from build123d import *
from build123d import SkipClean  # not in build123d's __all__

# Parameters (mm, degrees)
F0_W                   = 3
F0_H                   = 25.3
F0_W_2                 = 30.5
F1_DEPTH               = 3
F2_DEPTH               = 5
F3_R                   = 1.35
F4_DEPTH               = 500
F7_SIZE                = 5
F8_R                   = 1.35
F9_DEPTH               = 1
F10_W                  = 15
F10_H                  = 15
F11_DEPTH              = 3
F12_W                  = 4
F12_H                  = 5
F13_DEPTH              = 3
F12_W_2                = 4.5
F12_H_2                = 5.5
F14_DEPTH              = 25
F15_DEPTH              = 5
F16_R                  = 3.75
F17_DEPTH              = 2
F20_D                  = 3
F20_DEPTH              = 3
F20_CBORE_D            = 3
F20_CBORE_DEPTH        = 3
F20_TIP                = 0.9012909285
F20_ON_F19_D           = 3
F20_ON_F19_DEPTH       = 3
F20_ON_F19_CBORE_D     = 3
F20_ON_F19_CBORE_DEPTH = 3
F20_ON_F19_TIP         = 0.9012909285
F21_SIZE               = 10
F22_DEPTH              = 1
F23_SIZE               = 4.99999


# Not quite as in the source:
# - a fillet or chamfer is up to 0.001 mm smaller than in the source, because OpenCascade refuses the exact size


with BuildPart() as f1:
    # F0 (on Top) → F1 (new body)
    with BuildSketch(Plane.XY):
        with Locations((16.75, 0)):
            Rectangle(F0_W, F0_H)
        Rectangle(F0_W_2, F0_H)
        with Locations((-16.75, 0)):
            Rectangle(F0_W, F0_H)
    extrude(amount=F1_DEPTH)

    # F0 (on Top) → F2 (join)
    with BuildSketch(Plane.XY):
        with Locations((16.75, 0)):
            Rectangle(F0_W, F0_H)
        with Locations((-16.75, 0)):
            Rectangle(F0_W, F0_H)
    extrude(amount=-F2_DEPTH)

    # F3 (on face) → F4 (cut, symmetric)
    with BuildSketch(Plane(origin=(15.25, 0, 0), x_dir=(0, -1, 0), z_dir=(-1, 0, 0))):
        with BuildLine():
            Line((12.65, -4.15), (12.65, -1.45))
            ThreePointArc((12.65, -1.45), (11.3, -2.8), (12.65, -4.15))
        make_face()
        with Locations((-4.35, -2.8)):
            Circle(F3_R)
    extrude(amount=F4_DEPTH, both=True, mode=Mode.SUBTRACT)

    # F6: F1 across plane


with BuildPart() as f1_1:
    add(f1.part, clean=False)
    with SkipClean():  # cleaning this boolean's faces spoils the solid; the shape is the same uncleaned
        add(f1.part.mirror(Plane.XZ.offset(12.65)), clean=False)

    # F7
    f7_edges = [f1_1.edges().sort_by_distance(p)[0] for p in [
        (-16.75, 12.65, -5),
        (16.75, 12.65, -5),
        (16.75, -37.95, -5),
        (-16.75, -37.95, -5),
    ]]
    chamfer(f7_edges, length=F7_SIZE)

    # F8 (on face) → F9 (cut)
    with BuildSketch(Plane(origin=(-18.25, 0, 0), x_dir=(0, -1, 0), z_dir=(-1, 0, 0))):
        with BuildLine():
            Line((12.65, 0), (-12.65, 0))
            Line((-12.65, 0), (-7.65, -5))
            Line((-7.65, -5), (12.65, -5))
            Line((12.65, -5), (12.65, -4.15))
            ThreePointArc((12.65, -4.15), (11.3, -2.8), (12.65, -1.45))
            Line((12.65, -1.45), (12.65, 0))
        make_face()
        with Locations((-4.35, -2.8)):
            Circle(F8_R, mode=Mode.SUBTRACT)
        with BuildLine():
            Line((37.95, 0), (12.65, 0))
            Line((12.65, 0), (12.65, -1.45))
            ThreePointArc((12.65, -1.45), (14, -2.8), (12.65, -4.15))
            Line((12.65, -4.15), (12.65, -5))
            Line((12.65, -5), (32.95, -5))
            Line((32.95, -5), (37.95, 0))
        make_face()
        with Locations((29.65, -2.8)):
            Circle(F8_R, mode=Mode.SUBTRACT)
    extrude(amount=-F9_DEPTH, mode=Mode.SUBTRACT)

    # F10 (on Top) → F11 (join)
    with BuildSketch(Plane.XY):
        with Locations((-10.75, -45.45)):
            Rectangle(F10_W, F10_H)
        with Locations((-10.75, 20.15)):
            Rectangle(F10_W, F10_H)
    extrude(amount=F11_DEPTH)

    # F12 (on face) → F13 (join)
    with BuildSketch(Plane(origin=(0, 0, 0), x_dir=(1, 0, 0), z_dir=(0, 0, -1))):
        with Locations((-20.25, 50.45)):
            Rectangle(F12_W, F12_H)
    extrude(amount=-F13_DEPTH)

    # F12 (on face) → F14 (cut)
    with BuildSketch(Plane(origin=(0, 0, 0), x_dir=(1, 0, 0), z_dir=(0, 0, -1))):
        with Locations((-16, -24.9)):
            Rectangle(F12_W_2, F12_H_2)
    extrude(amount=-F14_DEPTH, mode=Mode.SUBTRACT)

    # F15 (add): faces of the model
    f15_faces = [f1_1.faces().sort_by_distance(p)[0] for p in [
        (-18.25, 0, 1.5),
        (-18.25, -25.3, 1.5),
        (-18.25, -42.95, 1.5),
        (-18.25, 17.4, 1.5),
        (-22.25, -50.45, 1.5),
        (-13.75, 24.9, 1.5),
    ]]
    extrude(f15_faces, amount=F15_DEPTH)

    # F16 (on face) → F17 (join)
    with BuildSketch(Plane(origin=(0, 0, 0), x_dir=(1, 0, 0), z_dir=(0, 0, -1))):
        with BuildLine():
            Line((-13.75, -22.15), (-18, -22.15))
            ThreePointArc((-18, -22.15), (-16.7185522073, -24.9728974477), (-13.75, -25.8665171868))
            Line((-13.75, -25.8665171868), (-13.75, -22.15))
        make_face()
        with BuildLine():
            ThreePointArc((-13.75, -25.8665171868), (-11.4271025523, -24.6185522073), (-10.5, -22.15))
            ThreePointArc((-10.5, -22.15), (-14.25, -18.4), (-18, -22.15))
            Line((-18, -22.15), (-13.75, -22.15))
            Line((-13.75, -22.15), (-13.75, -25.8665171868))
        make_face()
        with Locations((-14.25, 47.45)):
            Circle(F16_R)
    extrude(amount=F17_DEPTH)

    # F20
    with Locations(Plane(origin=(0, 0, -2), x_dir=(1, 0, 0), z_dir=(0, 0, -1))):
        with Locations((-14.25, 47.45)):
            CounterBoreHole(F20_D / 2, F20_CBORE_D / 2, F20_CBORE_DEPTH, depth=F20_DEPTH)
            with Locations((0, 0, -(F20_DEPTH + F20_TIP / 2))):  # 118° drill point
                Cone(0, F20_D / 2, F20_TIP, mode=Mode.SUBTRACT)

    # F20 on F19
    with Locations(Plane(origin=(0, 0, -2), x_dir=(1, 0, 0), z_dir=(0, 0, -1))):
        with Locations((-14.25, -22.15)):
            CounterBoreHole(F20_ON_F19_D / 2, F20_ON_F19_CBORE_D / 2, F20_ON_F19_CBORE_DEPTH, depth=F20_ON_F19_DEPTH)
            with Locations((0, 0, -(F20_ON_F19_DEPTH + F20_ON_F19_TIP / 2))):  # 118° drill point
                Cone(0, F20_ON_F19_D / 2, F20_ON_F19_TIP, mode=Mode.SUBTRACT)

    # F21
    f21_edges = [f1_1.edges().sort_by_distance(p)[0] for p in [
        (-3.25, 27.65, 1.5),
        (-3.25, -52.95, 1.5),
    ]]
    chamfer(f21_edges, length=F21_SIZE)

    # F22 (cut): a face of the model
    f22_faces = [f1_1.faces().sort_by_distance(p)[0] for p in [
        (18.25, -12.65, -0.7538732148),
    ]]
    extrude(f22_faces, amount=-F22_DEPTH, mode=Mode.SUBTRACT)

    # F23 (size 5 in the source; OpenCascade refuses exactly that, so slightly less here)
    f23_edges = [f1_1.edges().sort_by_distance(p)[0] for p in [
        (-3.25, -37.95, 1.5),
        (-3.25, 12.65, 1.5),
    ]]
    chamfer(f23_edges, length=F23_SIZE)


solid = f1_1.part
Model file for the job. Use its own axes, mm. A direction names the side the tool comes from. Give positions to 0.01 mm unless a question says otherwise; leave off trailing zeros. Write each loop counter-clockwise with the first axis right and the second up, starting at its lowest first coordinate (ties: lowest second). Pieces come first, ordered by that corner, then holes. Notation, with made-up numbers: M -6.75,63 L 40.25,63 A25 cw 40.25,81 Z; hole C 85,-37 d8. An arc over 180 degrees is marked long. One line per item, written item: value. Start each with the question number.
Q1. Saw through at C-C, the plane y = -27. Write the cut outline in (x, z), plus the area to 4 significant figures.
Q2. Drop flat-ended pins along their axis: pin 1 Ø3 at (y, z) = (17.5, 0) entering from +X; pin 2 Ø1.5 at (x, z) = (10, 1) entering from +Y; pin 3 Ø1.5 at (y, z) = (25, 2) entering from -X. Give the stop position or say it passes through.
Q3. Probe probe 1 along Y at (x, z) = (-14.25, -0.4); probe 2 along X at (y, z) = (-1, -0.5); probe 3 along Y at (x, z) = (-14.25, 0.1). List the from-to ranges inside material, lowest first. Write a range as [from, to].
Q4. 3-axis set-ups, long thin cutter, end or side, ignore diameter. For faces 4 (the flat face through (-16.26, 10.12, -2.53)), 5 (the flat face through (-14, 24, -2)), 6 (the flat face through (-18.75, 25, 1)): which of +Z, -Z, +X, -X, +Y, -Y reach the whole face in a straight line?
Q5. Saw through at D-D, the plane y = -45. Write the cut outline in (x, z), plus the area to 3 significant figures.
Q6. Saw through at B-B, the plane x = -12. Write the cut outline in (y, z), plus the area to 3 significant figures.
Q7. Two-plate mould, pull along Z, no slides. Class faces 1 (the cylindrical face through (-16.26, -31, -2.74)), 2 (the flat face through (16, -13, -5)), 3 (the flat face through (-0.8, 15.2, 1.5)): +Z half, -Z half, draft (parallel to the pull), parting line (faces both ways), or undercut.
Q8. Saw through at A-A, the plane y = 4.35. Write the cut outline in (x, z).
Output values:
1. outline: M -23.25,0 L -17.25,0 L -17.25,-5 L -15.25,-5 L -15.25,0 L 15.25,0 L 15.25,-5 L 17.25,-5 L 17.25,3 L -23.25,3 Z
1. area: 141.5 mm²
2. pin 1: stops at x = -1.6
2. pin 2: stops at y = 12.65
2. pin 3: stops at x = -18.75
3. probe 1: y = [-51.2, -48.95], [-45.95, -43.7], [18.4, 20.65], [23.65, 25.9]
3. probe 2: x = [-17.25, -15.25], [15.25, 17.25]
3. probe 3: y = [-52.95, -48.95], [-45.95, 20.65], [23.65, 27.65]
4. face 4: -Z, +X, -X
4. face 5: -Z, +X, -X, +Y
4. face 6: +Z, -Z, -X, +Y
5. outline: M -23.25,0 L -17.09,0 L -17.09,-2 L -11.41,-2 L -11.41,0 L -5.3,0 L -5.3,3 L -23.25,3 Z
5. area: 65.2 mm²
6. outline: M -51.7,0 L -50.45,0 L -50.45,-2 L -44.45,-2 L -44.45,0 L 19.15,0 L 19.15,-2 L 25.15,-2 L 25.15,0 L 26.4,0 L 26.4,3 L -51.7,3 Z
6. area: 258 mm²
7. face 1: undercut
7. face 2: -Z half
7. face 3: draft
8. outline: M -23.25,0 L -17.25,0 L -17.25,-1.45 L -15.25,-1.45 L -15.25,0 L 15.25,0 L 15.25,-1.45 L 17.25,-1.45 L 17.25,3 L -23.25,3 Z; M -17.25,-5 L -15.25,-5 L -15.25,-4.15 L -17.25,-4.15 Z; M 15.25,-5 L 17.25,-5 L 17.25,-4.15 L 15.25,-4.15 Z
